Drawing for the job (mm, zero at the part's lowest x, y, z). A direction names the side the tool comes from. Give positions to 0.01 mm unless a question says otherwise; leave off trailing zeros. Loops run counter-clockwise (first coordinate to the right, second up) from the corner with the lowest first, then second, coordinate; pieces in that order, holes last. Notation, with made-up numbers: (57, -18) - (73, -18) arc R18 ccw to (73, -11) - close; hole circle Ø8 at (-10.5, 35.25). An arc over 180 degrees is marked (long way). Return JSON: item names as keys, results as strings. Group by question number.
1) Drill centre lines: probe 1 along Y at (x, z) = (43, 31); probe 2 along Y at (x, z) = (75.5, 42); probe 3 along X at (y, z) = (78.5, 27.5). Where is each one in solid material? Low to high. Write a range as from..to.
2) Slice it at A-A (x = 52). List the corners of the cut face in (y, z).
3) Slice it at C-C (y = 81.5). List the corners of the cut face in (x, z).
4) Mould opens along Y. For the marked faces 1, 2 and 3 say: released by +Y, released by -Y, zero draft, split by the parting line, or undercut.
5) Slice it at B-B (z = 36). List the corners of the cut face in (x, y).
6) Drop flat-ended pins along their axis: pin 1 (4.5 mm diameter, centred on x = 45, z = 25.5, fed in from -Y); pin 2 (7.5 mm diameter, centred on y = 80.5, z = 23, fed in from +X); pin 3 (10 mm diameter, centred on x = 62.5, y = 35.5, fed in from -Z); pin 4 (10 mm diameter, centred on y = 28, z = 27, fed in from -X). Give the stop position or say it passes through.
7) 3-axis set-ups, long thin cutter, end or side, ignore diameter. For the marked faces 4, 5, 6 and 7: which of +Z, -Z, +X, -X, +Y, -Y reach the whole face in a straight line?
8) Slice it at D-D (x = 73). List the corners of the cut face in (y, z), and give its area (3 significant figures).
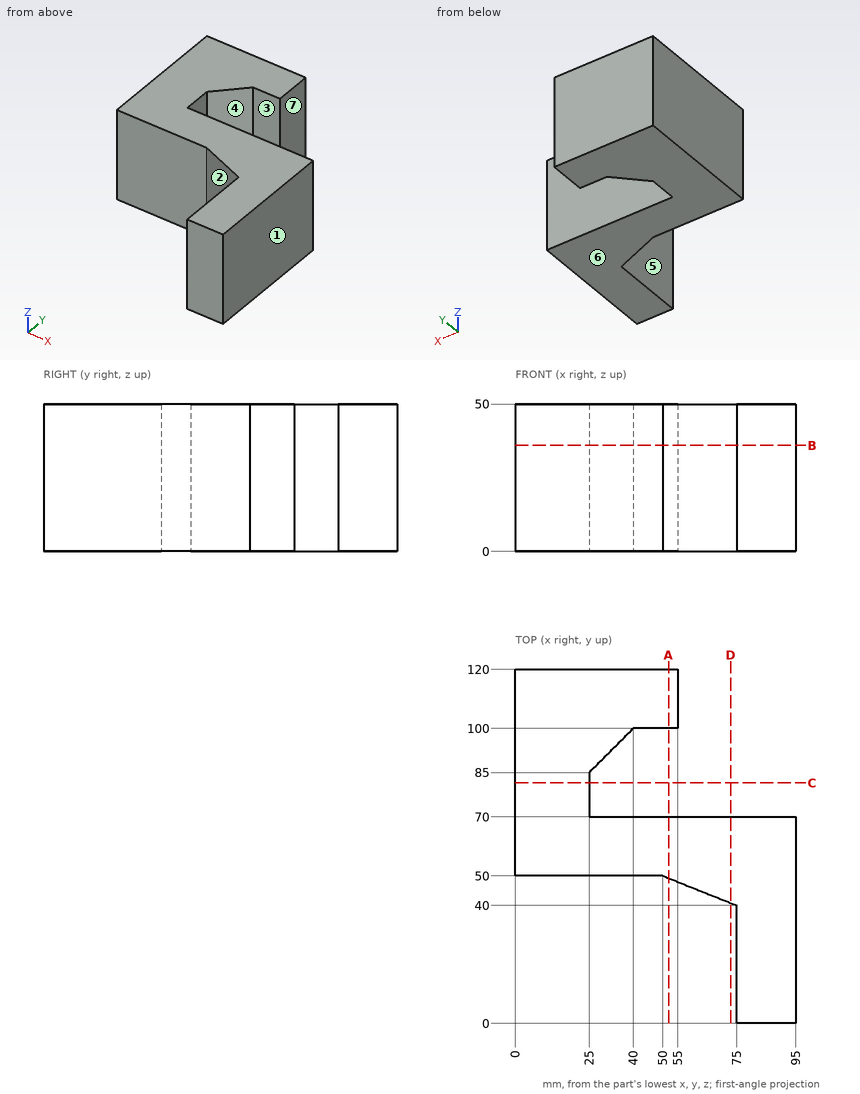
Results:
{
 "1": {"probe 1": "50..70, 100..120", "probe 2": "0..70", "probe 3": "0..25"},
 "2": {"outline": "(49.2, 0) - (70, 0) - (70, 50) - (49.2, 50) - close; (100, 0) - (120, 0) - (120, 50) - (100, 50) - close"},
 "3": {"outline": "(0, 0) - (25, 0) - (25, 50) - (0, 50) - close"},
 "4": {"face 1": "zero draft", "face 2": "released by -Y", "face 3": "undercut"},
 "5": {"outline": "(0, 50) - (50, 50) - (75, 40) - (75, 0) - (95, 0) - (95, 70) - (25, 70) - (25, 85) - (40, 100) - (55, 100) - (55, 120) - (0, 120) - close"},
 "6": {"pin 1": "y = 50", "pin 2": "x = 25", "pin 3": "through", "pin 4": "x = 75"},
 "7": {"face 4": "+Z, -Z, +X", "face 5": "+Z, -Z, -X, -Y", "face 6": "-Z, +X, -X, +Y, -Y", "face 7": "+Z, -Z, +X, +Y"},
 "8": {"outline": "(40.8, 0) - (70, 0) - (70, 50) - (40.8, 50) - close", "area": "1,460 mm2"}
}
